Source: three-view drawing plus pictorial views. Frame: mm from the lowest corner of the part. A direction names the side the tool comes from. Give positions to 0.01 mm unless a question says otherwise; leave off trailing zeros. Loops run counter-clockwise (first coordinate to the right, second up) from the corner with the lowest first, then second, coordinate; pieces in that order, holes last.
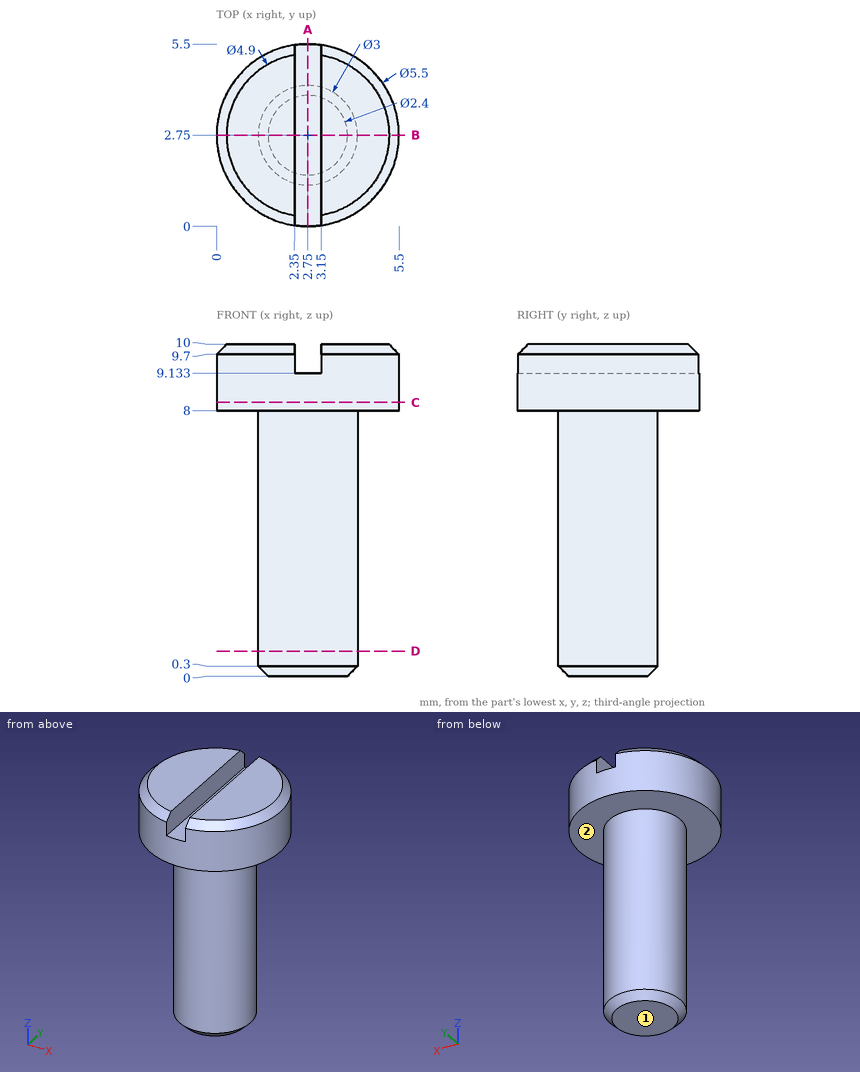
(1) Cut plane D-D (z = 0.75). Return the cut outline in (x, y).
Values follow:
outline: circle Ø3 at (2.75, 2.75)
(2) Cut plane C-C (z = 8.25). Return the cut outline in (x, y).
Values follow:
outline: circle Ø5.5 at (2.75, 2.75)
(3) Cut plane B-B (y = 2.75). Return the cut outline in (x, z).
Values follow:
outline: (0, 8) - (1.25, 8) - (1.25, 0.3) - (1.55, 0) - (3.95, 0) - (4.25, 0.3) - (4.25, 8) - (5.5, 8) - (5.5, 9.7) - (5.2, 10) - (3.15, 10) - (3.15, 9.13) - (2.35, 9.13) - (2.35, 10) - (0.3, 10) - (0, 9.7) - close
(4) Cut plane A-A (x = 2.75). Return the cut outline in (y, z).
Values follow:
outline: (0, 8) - (1.25, 8) - (1.25, 0.3) - (1.55, 0) - (3.95, 0) - (4.25, 0.3) - (4.25, 8) - (5.5, 8) - (5.5, 9.13) - (0, 9.13) - close
(5) Reachability of the marked faces 1 and 2 from +Z, -Z, +X, -X, +Y, -Y: full face, straight path, thin tool, end or side. Return the list, or none.
Values follow:
face 1: -Z, +X, -X, +Y, -Y
face 2: -Z
(6) Pin query (flat end, axial travel): pin 1 Ø1 at (x, z) = (1, 7) entering from +Y; pin 2 Ø1 at (y, z) = (2, 9.5) entering from -X. Return the tip coordinate at first contact, or that it passes through.
Values follow:
pin 1: stops at y = 3.58
pin 2: stops at x = 0.01
(7) Ray query, probe 1 along Z at (x, y) = (2.55, 4.5); probe 2 along Z at (x, y) = (2.05, 0.9); probe 3 along Y at (x, z) = (2.85, 7). Return the intervals inside material, ascending.
Values follow:
probe 1: z = 8 to 9.13
probe 2: z = 8 to 10
probe 3: y = 1.25 to 4.25
